from build123d import *

# Parameters (mm, degrees)
BASE_FLANGE1_DEPTH   = 1.5875
EDGE_FLANGE1_DEPTH   = 17.78
M4_CLEARANCE_HOLE1_D = 4.5
FILLET1_R            = 1.27


# Sheet-metal steps are written as plain solids
with BuildPart() as part:
    # Sketch1 → Base-Flange1 (new body)
    with BuildSketch(Plane(origin=(0, 0, 0), x_dir=(1, 0, 0), z_dir=(0, 1, 0))):
        with BuildLine():
            Line((-8.89, -9.069614104), (-8.89, -28.119614104))
            Line((-8.89, -28.119614104), (8.89, -28.119614104))
            Line((8.89, -28.119614104), (8.89, -9.069614104))
            ThreePointArc((8.89, -9.069614104), (0, -12.7), (-8.89, -9.069614104))
        make_face()
    extrude(amount=-BASE_FLANGE1_DEPTH)

    # Edge-Flange1 section (across the edge) → Edge-Flange1 (add)
    with BuildSketch(Plane(origin=(-8.89, 0, 29.389614104), x_dir=(0, 0, -1), z_dir=(1, 0, 0))):
        with BuildLine():
            Line((-1.5875, 1), (-1.5875, 57.15))
            Line((-1.5875, 57.15), (0, 57.15))
            Line((0, 57.15), (0, 1))
            ThreePointArc((0, 1), (0.292893219, 0.292893219), (1, 0))
            Line((1, 0), (1.27, 0))
            Line((1.27, 0), (1.27, -1.5875))
            Line((1.27, -1.5875), (1, -1.5875))
            ThreePointArc((1, -1.5875), (-0.829638796, -0.829638796), (-1.5875, 1))
        make_face()
    extrude(amount=EDGE_FLANGE1_DEPTH)

    # M4 Clearance Hole1 (through all)
    with Locations(Plane(origin=(0, 0, 29.389614104), x_dir=(-1, 0, 0), z_dir=(0, 0, -1))):
        with Locations((0, 46.524999898), (0, 11.625)):
            Hole(M4_CLEARANCE_HOLE1_D / 2)

    # Fillet1
    fillet1_edges = [part.edges().sort_by_distance(p)[0] for p in [
        (-8.89, 57.15, 30.183364104),
        (8.89, 57.15, 30.183364104),
        (8.89, -0.79375, 9.069614104),
        (-8.89, -0.79375, 9.069614104),
    ]]
    fillet(fillet1_edges, radius=FILLET1_R)


solid = part.part
For this review, take the finished solid that the model builds, in its own axes (mm). A direction names the side the tool comes from. Give positions to 0.01 mm unless a question says otherwise; leave off trailing zeros. Loops run counter-clockwise (first coordinate to the right, second up) from the corner with the lowest first, then second, coordinate; pieces in that order, holes last.
Item 1: For line 1 along Y through (x, z) = (0, 29.9) (3 decimals); line 2 along Y through (x, z) = (0, 30.4) (3 decimals); line 3 along Z through (x, y) = (7, 11.5), list the stretches that pass through material, from the lowest coordinate up.
Item 2: Tool access review of faces 4 (the cylindrical face through (8.528, 56.768, 30.172)), 5 (the flat face through (0, 29, 29.39)): name each direction out of +Z, -Z, +X, -X, +Y, -Y from which nothing blocks a thin tool from reaching the whole face with its end or side.
Item 3: Draft analysis for pull direction X (two halves, no side actions). For faces 1 (the cylindrical face through (-8.528, 56.768, 30.172)), 2 (the cylindrical face through (0.1, -0.8, 12.7)), 3 (the flat face through (0, -1.588, 19)), state which applies: +X half, -X half, draft (parallel to the pull), parting line (faces both ways), or undercut.
Item 4: Take a section at A-A, the plane x = 0. Give the number of separate pieces and of enclosed holes in the cut face, and give its area (3 significant figures).
Item 5: Take a section at B-B, the plane y = 47.5. State the section outline as (x, z) points, and give its area (3 significant figures).
Item 6: Insertion check: pin 1 (1.5 mm diameter, centred on x = 0, y = 21, fed in from -Z); pin 2 (8 mm diameter, centred on y = 17, z = 24.5, fed in from -X). Each pin has a flat end and moves straight along its axis. Give the tip position at first contact, or say it passes through.
Item 7: Take a section at C-C, the plane z = 20. State the section outline as (x, y) points.
Calculated:
1. line 1: y = -1.101 to 9.375, 13.875 to 44.275, 48.775 to 57.15
1. line 2: y = -0.629 to 9.375, 13.875 to 44.275, 48.775 to 57.15
1. line 3: z = 29.39 to 30.98
2. face 4: +Z, -Z, +X, +Y
2. face 5: -Z, +X, -X, +Y
3. face 1: -X half
3. face 2: undercut
3. face 3: draft
4. separate pieces: 3
4. enclosed holes: 0
4. area: 104 mm2
5. outline: (-8.89, 29.39) - (-2.03, 29.39) - (-2.03, 30.98) - (-8.89, 30.98) - close; (2.03, 29.39) - (8.89, 29.39) - (8.89, 30.98) - (2.03, 30.98) - close
5. area: 21.8 mm2
6. pin 1: stops at z = 29.39
6. pin 2: passes through
7. outline: (-8.89, -1.59) - (8.89, -1.59) - (8.89, 0) - (-8.89, 0) - close
